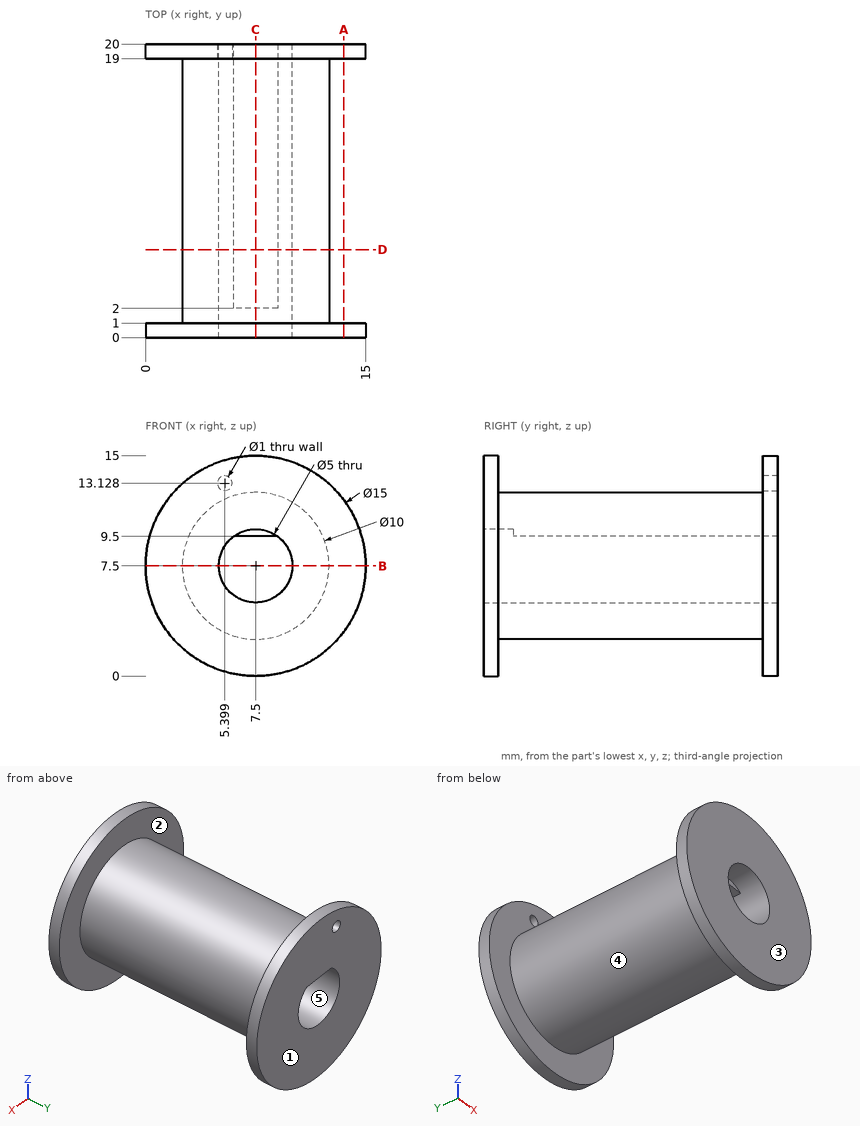
Geometry: see drawing. Coordinates: mm, zero at the bounding-box minimum. A direction names the side the tool comes from. Coordinates: 2 decimals unless noted, no trailing zeros. Loops run counter-clockwise (first coordinate to the right, second up) from the corner with the lowest first, then second, coordinate; pieces in that order, holes last. Notation, with made-up numbers: M -19.5,32.25 L 6.5,32.25 A19 cw 6.5,45.25 Z; hole C 65.5,10.5 d8. An arc over 180 degrees is marked long. Answer in a Markdown table with one row per item.
1. Section D-D, the plane y = 6. Output: boundary loops of the cut face in (x, z), then the cut area to 3 significant figures.
Response:
| item | result |
|---|---|
| outline | C 7.5,7.5 d10; hole M 6,9.5 A2.5 ccw long 9,9.5 Z |
| area | 59.9 mm2 |
2. Material intervals for line 1 (Z direction, x = 7.5, y = 7.25); line 2 (Y direction, x = 12.5, z = 6.75); line 3 (X direction, y = 13.5, z = 7.5), sorted ascending.
Response:
| item | result |
|---|---|
| line 1 | z = 2.5 to 5, 9.5 to 12.5 |
| line 2 | y = 0 to 1, 19 to 20 |
| line 3 | x = 2.5 to 5, 10 to 12.5 |
3. Section B-B, the plane z = 7.5. Output: boundary loops of the cut face in (x, y).
Response:
| item | result |
|---|---|
| outline | M 0,0 L 5,0 L 5,20 L 0,20 L 0,19 L 2.5,19 L 2.5,1 L 0,1 Z; M 10,0 L 15,0 L 15,1 L 12.5,1 L 12.5,19 L 15,19 L 15,20 L 10,20 Z |
4. Reachability of the marked faces 1 and 2 from +Z, -Z, +X, -X, +Y, -Y: full face, straight path, thin tool, end or side. Return the list, or none.
Response:
| item | result |
|---|---|
| face 1 | +Z, -Z, +X, -X, +Y |
| face 2 | none |
5. First-contact query: pin 1 (4 mm diameter, centred on y = 9, z = 5.5, fed in from +X); pin 2 (3 mm diameter, centred on y = 3, z = 12.5, fed in from -X); pin 3 (1.5 mm diameter, centred on x = 10, y = 5, fed in from -Z). Flat tips, straight axial feed; report the tip coordinate or a pass-through.
Response:
| item | result |
|---|---|
| pin 1 | stops at x = 12.5 |
| pin 2 | stops at x = 3.93 |
| pin 3 | stops at z = 2.82 |
6. Section A-A, the plane x = 13.5. Output: boundary loops of the cut face in (y, z).
Response:
| item | result |
|---|---|
| outline | M 0,3 L 1,3 L 1,12 L 0,12 Z; M 19,3 L 20,3 L 20,12 L 19,12 Z |
7. Section C-C, the plane x = 7.5. Output: boundary loops of the cut face in (y, z), then the cut area to 3 significant figures.
Response:
| item | result |
|---|---|
| outline | M 0,0 L 1,0 L 1,2.5 L 19,2.5 L 19,0 L 20,0 L 20,5 L 0,5 Z; M 0,10 L 2,10 L 2,9.5 L 20,9.5 L 20,15 L 19,15 L 19,12.5 L 1,12.5 L 1,15 L 0,15 Z |
| area | 119 mm2 |
8. Draft query along X for the marked faces 3, 4 and 5. Return one class per face: pulls with the +X half, pulls with the -X half, needs draft (parallel to the pull), parting line crosses it, or undercut.
Response:
| item | result |
|---|---|
| face 3 | needs draft |
| face 4 | parting line crosses it |
| face 5 | undercut |
